Check sheet for the modelled part. Datum: model origin and axes. Units: mm. Face numbers are marked on the shaded views. Give positions to 0.01 mm unless a question says otherwise; leave off trailing zeros. Order: outer loops, then holes, each group sorted by start corner. A loop starts at its lowest first (then second) coordinate and runs counter-clockwise, first axis right, second up. Notation, with made-up numbers: (78, -33) -> (90, -33) arc R6 cw to (90, -22) -> close; hole circle Ø8 at (30.25, -32). An arc over 180 degrees is marked (long way). Answer in a Markdown table with one row per item. Add a question column.
(1) Thickness scan on L1, parallel to X at y = -9, z = 0.55; L2, parallel to Y at x = 1.5, z = 1.4; L3, parallel to X at y = -17, z = 2.9. Record the ranges inside material, lowest first. Write a range as [from, to].
(2) Cross-section at B-B (y = 18.5). Record the cut outline in (x, z), then the cut area to 3 significant figures.
(3) Cross-section at C-C (x = -21). Record the cut outline in (y, z).
(4) Cross-section at D-D (z = 1.1). State how many separate pieces and enclosed holes the cut face has, then the cut area to 3 significant figures.
(5) Cross-section at A-A (x = 0). Record the cut outline in (y, z), then the cut area to 3 significant figures.
(6) Go/stop test with flat-tipped pins: pin 1 (3 mm diameter, centred on x = -19, z = 1, fed in from +Y); pin 2 (3 mm diameter, centred on y = -12, z = 3.5, fed in from -X); pin 3 (1 mm diameter, centred on y = -16, z = 1, fed in from -X). Record where each tip stops, or that it passes through.
(7) Release check for a two-part mould opening along Y. For the marked faces 1, 2 and 3 record: released by +Y, released by -Y, zero draft, split by the parting line, or undercut.
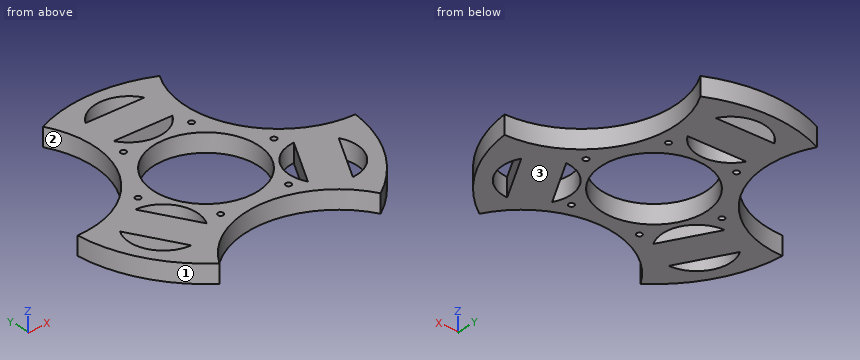
```python
from build123d import *

# Parameters (mm, degrees)
F0_R     = 0.762
F0_R_2   = 14.3129
F1_DEPTH = 5.08


with BuildPart() as f1:
    # F0 (on Top) → F1 (new body)
    with BuildSketch(Plane.XY):
        with BuildLine():
            ThreePointArc((37.814819, -4.652899), (16.218364, 8.71367), (16.993927, 34.100094))
            ThreePointArc((16.993927, 34.100094), (1.190918, 38.081383), (-14.829981, 35.095322))
            ThreePointArc((-14.829981, 35.095322), (-15.650884, 9.718876), (-38.032383, -2.268884))
            ThreePointArc((-38.032383, -2.268884), (-33.588812, -17.983373), (-22.974289, -30.393948))
            ThreePointArc((-22.974289, -30.393948), (-0.586685, -18.405835), (20.992008, -31.795371))
            ThreePointArc((20.992008, -31.795371), (32.384242, -20.071643), (37.814819, -4.652899))
        make_face()
        with BuildLine():
            ThreePointArc((-22.674204, -21.077907), (-30.514378, -16.211576), (-30.292149, -6.986604))
            Line((-30.292149, -6.986604), (-22.674204, -21.077907))
        make_face(mode=Mode.SUBTRACT)
        with Locations((-9.776836, -15.761217)):
            Circle(F0_R, mode=Mode.SUBTRACT)
        with BuildLine():
            ThreePointArc((-22.077247, -2.545519), (-14.247146, -7.417295), (-14.459302, -16.636821))
            Line((-14.459302, -16.636821), (-22.077247, -2.545519))
        make_face(mode=Mode.SUBTRACT)
        with Locations((8.761197, -16.347597)):
            Circle(F0_R, mode=Mode.SUBTRACT)
        with BuildLine():
            ThreePointArc((12.561953, -18.186712), (12.756508, -9.109725), (20.600149, -4.537325))
            Line((20.600149, -4.537325), (12.561953, -18.186712))
        make_face(mode=Mode.SUBTRACT)
        with Locations((18.538033, -0.58638)):
            Circle(F0_R, mode=Mode.SUBTRACT)
        with BuildLine():
            Line((20.866679, -23.077409), (28.904875, -9.428021))
            ThreePointArc((28.904875, -9.428021), (28.701601, -18.499874), (20.866679, -23.077409))
        make_face(mode=Mode.SUBTRACT)
        with Locations((-18.538033, 0.58638)):
            Circle(F0_R, mode=Mode.SUBTRACT)
        with Locations((-8.761197, 16.347597)):
            Circle(F0_R, mode=Mode.SUBTRACT)
        Circle(F0_R_2, mode=Mode.SUBTRACT)
        with BuildLine():
            ThreePointArc((8.55484, 20.415134), (0.392702, 16.148838), (-7.463453, 20.955355))
            Line((-7.463453, 20.955355), (8.55484, 20.415134))
        make_face(mode=Mode.SUBTRACT)
        with Locations((9.776836, 15.761217)):
            Circle(F0_R, mode=Mode.SUBTRACT)
        with BuildLine():
            Line((8.8691, 29.733366), (-7.149193, 30.273587))
            ThreePointArc((-7.149193, 30.273587), (1.013642, 34.560545), (8.8691, 29.733366))
        make_face(mode=Mode.SUBTRACT)
    extrude(amount=F1_DEPTH)


solid = f1.part
```
Answer below:
| question | item | result |
|---|---|---|
| 1 | L1 | x = [-37.02, -31.2], [-29.2, -18.59], [-13.57, -11.13], [11.13, 12.82], [17.97, 37.02] |
| 1 | L2 | y = [-18.56, -14.23], [14.23, 16.18], [20.65, 29.98], [34.53, 38.07] |
| 1 | L3 | x = [-34.1, -30.04], [-24.88, 8.37], [9.15, 12.03], [13.26, 24.45], [29.41, 34.1] |
| 2 | outline | (-12.25, 0) -> (-5.5, 0) -> (-5.5, 5.08) -> (-12.25, 5.08) -> close; (6.91, 0) -> (13.29, 0) -> (13.29, 5.08) -> (6.91, 5.08) -> close |
| 2 | area | 66.7 mm² |
| 3 | outline | (-27.64, 0) -> (-4.54, 0) -> (-4.54, 5.08) -> (-27.64, 5.08) -> close; (-2.65, 0) -> (3.58, 0) -> (3.58, 5.08) -> (-2.65, 5.08) -> close |
| 4 | separate pieces | 1 |
| 4 | enclosed holes | 13 |
| 4 | area | 1,780 mm² |
| 5 | outline | (-18.43, 0) -> (-14.31, 0) -> (-14.31, 5.08) -> (-18.43, 5.08) -> close; (14.31, 0) -> (16.17, 0) -> (16.17, 5.08) -> (14.31, 5.08) -> close; (20.7, 0) -> (30.03, 0) -> (30.03, 5.08) -> (20.7, 5.08) -> close; (34.54, 0) -> (38.1, 0) -> (38.1, 5.08) -> (34.54, 5.08) -> close |
| 5 | area | 95.8 mm² |
| 6 | pin 1 | stops at y = 7.12 |
| 6 | pin 2 | stops at x = -36.62 |
| 6 | pin 3 | stops at x = -34.8 |
| 7 | face 1 | released by -Y |
| 7 | face 2 | undercut |
| 7 | face 3 | zero draft |
